Verification items for this drawing (mm, ordinates from the low corner). A direction names the side the tool comes from. Round coordinates to 2 decimals unless told otherwise and drop trailing zeros. Order: outer loops, then holes, each group sorted by start corner. A loop starts at its lowest first (then second) coordinate and runs counter-clockwise, first axis right, second up. Notation, with made-up numbers: (-18.75, 3) -> (25.25, 3) arc R17 ccw to (25.25, 20) -> close; hole circle Ø6 at (8.25, -30.5). An arc over 180 degrees is marked (long way). Put each result on its own line as item: value.
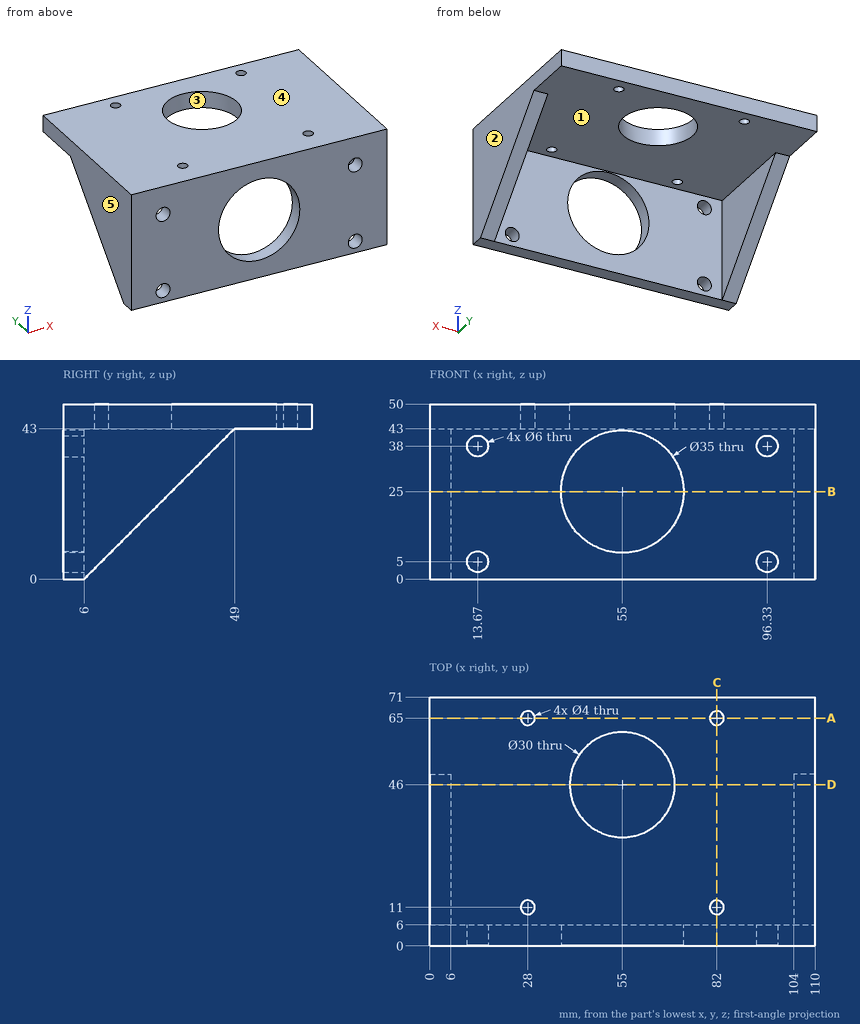
Item 1: Section check A-A on y = 65. Record the boundary of the cut face in (x, z), then the cut area to 3 significant figures.
Check sheet entries:
outline: (0, 43) -> (26, 43) -> (26, 50) -> (0, 50) -> close; (30, 43) -> (80, 43) -> (80, 50) -> (30, 50) -> close; (84, 43) -> (110, 43) -> (110, 50) -> (84, 50) -> close
area: 714 mm^2
Item 2: Tool access check on the marked faces 1 and 2. Record the directions out of +Z, -Z, +X, -X, +Y, -Y that give a thin tool (end or side, any length) a straight path to the whole face; none if there is none.
Check sheet entries:
face 1: -Z, +Y
face 2: +Z, -Z, +X, +Y, -Y
Item 3: Section check C-C on x = 82. Record the boundary of the cut face in (y, z).
Check sheet entries:
outline: (0, 0) -> (6, 0) -> (6, 43) -> (9, 43) -> (9, 50) -> (0, 50) -> close; (13, 43) -> (63, 43) -> (63, 50) -> (13, 50) -> close; (67, 43) -> (71, 43) -> (71, 50) -> (67, 50) -> close
Item 4: Gauge pin test, flat ends, axial feed: pin 1 Ø3.5 at (x, y) = (82, 11) entering from -Z (1 decimal); pin 2 Ø5 at (x, y) = (97.5, 27) entering from -Z; pin 3 Ø7 at (x, z) = (13.67, 38) entering from +Y. Record the tip position at first contact, or that the pin passes through.
Check sheet entries:
pin 1: passes through
pin 2: stops at z = 43
pin 3: stops at y = 6
Item 5: Release check for a two-part mould opening along X. For the marked faces 3, 4 and 5 record: +X half, -X half, draft (parallel to the pull), parting line (faces both ways), or undercut.
Check sheet entries:
face 3: undercut
face 4: draft
face 5: -X half
Item 6: Section check D-D on y = 46. Record the boundary of the cut face in (x, z), then the cut area to 3 significant figures.
Check sheet entries:
outline: (0, 40) -> (6, 40) -> (6, 43) -> (40, 43) -> (40, 50) -> (0, 50) -> close; (70, 43) -> (104, 43) -> (104, 40) -> (110, 40) -> (110, 50) -> (70, 50) -> close
area: 596 mm^2
Item 7: Section check B-B on z = 25. Record the boundary of the cut face in (x, y).
Check sheet entries:
outline: (0, 0) -> (37.5, 0) -> (37.5, 6) -> (6, 6) -> (6, 31) -> (0, 31) -> close; (72.5, 0) -> (110, 0) -> (110, 31) -> (104, 31) -> (104, 6) -> (72.5, 6) -> close
Item 8: Material ranges on L1, parallel to X at y = 2.6, z = 5; L2, parallel to Y at x = 28, z = 46.25; L3, parallel to X at y = 1.85, z = 25, recorded low to high. Write a range as [from, to].
Check sheet entries:
L1: x = [0, 10.67], [16.67, 93.33], [99.33, 110]
L2: y = [0, 9], [13, 63], [67, 71]
L3: x = [0, 37.5], [72.5, 110]
